Geometry check sheet. Reference: drawing and pictorial views, mm from the part's lowest x, y, z. Give positions to 0.01 mm unless a question says otherwise; leave off trailing zeros. Order: outer loops, then holes, each group sorted by start corner. A loop starts at its lowest first (then second) coordinate and runs counter-clockwise, first axis right, second up. Notation, with made-up numbers: (-8.5, 19.5) - (28.5, 19.5) arc R18 cw to (28.5, 36.5) - close; hole circle Ø6 at (-36.5, -35.5). An arc over 180 degrees is marked (long way). Answer in a Markdown table with one row per item.
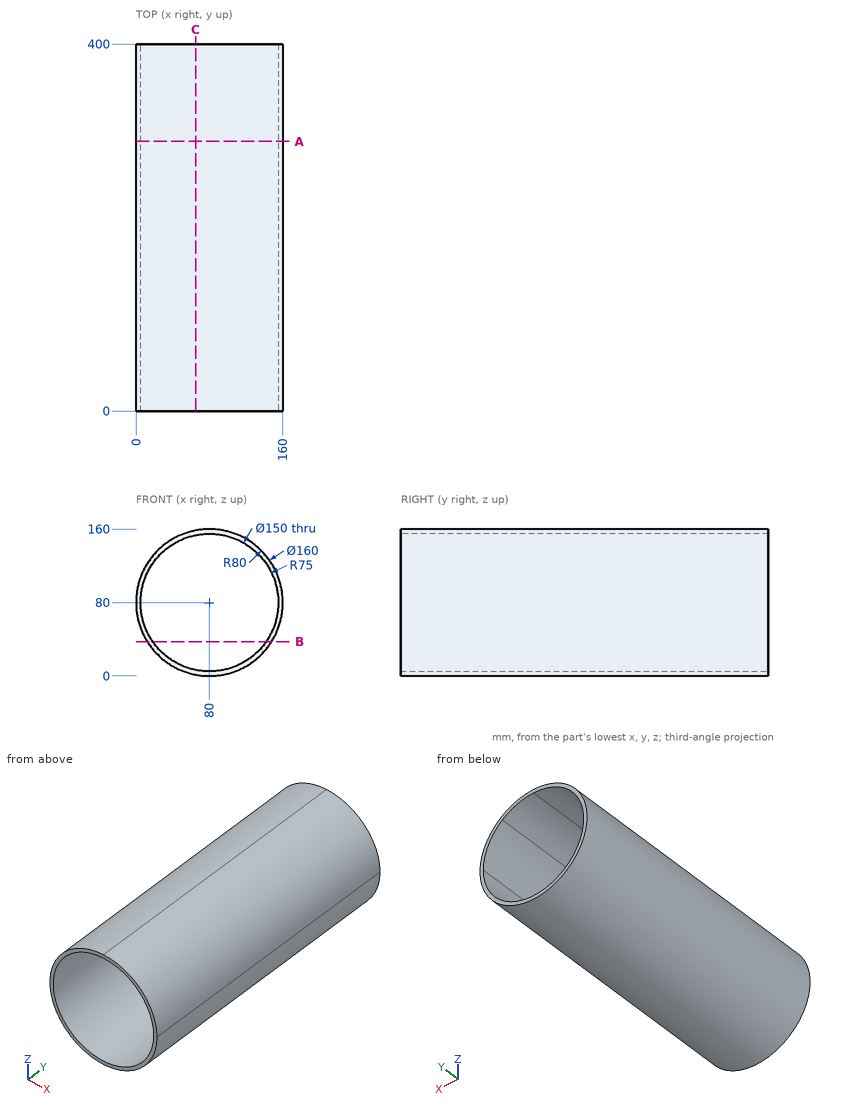
(1) Cross-section at B-B, the plane z = 37.5. Record the cut outline in (x, y).
Geometry says:
| item | result |
|---|---|
| outline | (12.22, 0) - (18.2, 0) - (18.2, 400) - (12.22, 400) - close; (141.8, 0) - (147.78, 0) - (147.78, 400) - (141.8, 400) - close |
(2) Thickness scan on L1, parallel to Z at x = 80, y = 101; L2, parallel to Z at x = 49.5, y = 330. Record the ranges inside material, lowest first.
Geometry says:
| item | result |
|---|---|
| L1 | 0 to 5, 155 to 160 |
| L2 | 6.04 to 11.48, 148.52 to 153.96 |
(3) Cross-section at C-C, the plane x = 65. Record the cut outline in (y, z).
Geometry says:
| item | result |
|---|---|
| outline | (0, 1.42) - (400, 1.42) - (400, 6.52) - (0, 6.52) - close; (0, 153.48) - (400, 153.48) - (400, 158.58) - (0, 158.58) - close |
(4) Cross-section at A-A, the plane y = 294. Record the cut outline in (x, z), then the cut area to 3 significant figures.
Geometry says:
| item | result |
|---|---|
| outline | (80, 160) arc R80 ccw (long way) to (160, 80) arc R80 ccw to start; hole (80, 155) arc R75 ccw (long way) to (155, 80) arc R75 ccw to (126.59, 138.77) arc R75 ccw to start |
| area | 2,430 mm² |
(5) Gauge pin test, flat ends, axial feed: P1, Ø12, axis at y = 339, z = 134.5, coming from the -X side; P2, Ø10, axis at x = 65, y = 105.5, coming from the -Z side; P3, Ø10, axis at x = 90, y = 161, coming from the -Z side. Record the tip position at first contact, or that the pin passes through.
Geometry says:
| item | result |
|---|---|
| P1 | x = 16.38 |
| P2 | z = 0.63 |
| P3 | z = 0.16 |
